from build123d import *

# Parameters (mm, degrees)
ESBO_O1_W                = 7.874
ESBO_O1_H                = 2.794
RESSALTO_EXTRUS_O1_DEPTH = 3


with BuildPart() as part:
    # Esboço1 → Ressalto-extrusão1 (new body)
    with BuildSketch(Plane.XY):
        Polygon((17.5, -95), (35, -80), (35, -28.1), (32, -25.1), (32, -20.1), (35, -17.1), (35, 0), (0, 0), (0, -17.1), (3, -20.1), (3, -25.1), (0, -28.1), (0, -80), align=None)
        with BuildLine():
            ThreePointArc((5, -30.3), (4.7, -30), (5, -29.7))
            Line((5, -29.7), (30, -29.7))
            ThreePointArc((30, -29.7), (30.3, -30), (30, -30.3))
            Line((30, -30.3), (5, -30.3))
        make_face(mode=Mode.SUBTRACT)
        with Locations((17.5, -7.397)):
            Rectangle(ESBO_O1_W, ESBO_O1_H, mode=Mode.SUBTRACT)
    extrude(amount=RESSALTO_EXTRUS_O1_DEPTH)


solid = part.part
Design review of the part built by this model. Coordinates are the model's own, in mm. A direction names the side the tool comes from. Coordinates: 2 decimals unless noted, no trailing zeros. Write each loop counter-clockwise with the first axis right and the second up, starting at its lowest first coordinate (ties: lowest second). Pieces come first, ordered by that corner, then holes. Notation, with made-up numbers: (40, 86) -> (65, 86) arc R17 ccw to (65, 106) -> close; hole circle Ø11 at (26, -6.5). An arc over 180 degrees is marked (long way). Write each question's results on one line, items separated by ' | '. Start each with the question number.
(1) Tool access review of faces 4 (the face through (1.5, -26.6, 1.5)), 5 (the face through (18, -30.3, 1)), 6 (the face through (32, -23, 1)), 7 (the face through (18, 0, 1)), 8 (the face through (8.628, -87.395, 1.479)): name each direction out of +Z, -Z, +X, -X, +Y, -Y from which nothing blocks a thin tool from reaching the whole face with its end or side.
(2) Clearance check with flat-ended pins moving along their axes: P1, Ø0.9, axis at y = -22, z = 1, coming from the +X side; P2, Ø0.9, axis at x = 23, z = 1, coming from the -Y side. State where each tip first meets the part, or that it passes through.
(3) The part is to be moulded in two halves that separate along X. For faces 1 (the face through (35, -9, 1)), 2 (the face through (17, -29.7, 1)), 3 (the face through (3, -23, 1)), say which applies: pulls with the +X half, pulls with the -X half, needs draft (parallel to the pull), parting line crosses it, or undercut.
(4) Take a section at A-A on z = 1.8. Write out the cut boundary in (x, y), and give its area (3 significant figures).
(5) For line 1 along Y through (x, z) = (21, 1.5); line 2 along Y through (x, z) = (18.5, 0.6); line 3 along Y through (x, z) = (29, 2.15), list the stretches that pass through material, from the lowest coordinate up. Write a range as from..to.
Results found:
1) face 4: +Z, -Z, -X | face 5: +Z, -Z | face 6: +Z, -Z, +X | face 7: +Z, -Z, +X, -X, +Y | face 8: +Z, -Z, -X, -Y
2) P1: stops at x = 32 | P2: stops at y = -90.67
3) face 1: pulls with the +X half | face 2: undercut | face 3: pulls with the -X half
4) outline: (0, -80) -> (17.5, -95) -> (35, -80) -> (35, -28.1) -> (32, -25.1) -> (32, -20.1) -> (35, -17.1) -> (35, 0) -> (0, 0) -> (0, -17.1) -> (3, -20.1) -> (3, -25.1) -> (0, -28.1) -> close; hole (5, -30.3) -> (30, -30.3) arc R0.3 ccw to (30, -29.7) -> (5, -29.7) arc R0.3 ccw to start; hole (13.56, -8.79) -> (21.44, -8.79) -> (21.44, -6) -> (13.56, -6) -> close | area: 2,980 mm2
5) line 1: y = -92..-30.3, -29.7..-8.79, -6..0 | line 2: y = -94.14..-30.3, -29.7..-8.79, -6..0 | line 3: y = -85.14..-30.3, -29.7..0
